Could you check a few things on this model? Use its own coordinates, in mm. Give positions to 0.01 mm unless a question says otherwise; leave off trailing zeros. Write each loop counter-clockwise with the first axis right and the second up, starting at its lowest first coordinate (ties: lowest second). Pieces come first, ordered by that corner, then holes. Notation, with made-up numbers: M -21,29 L -9,29 A27 ccw -9,61 Z; hole C -15.75,61 d1. An arc over 180 degrees is marked long. Use one line per item in the form item = value.
from build123d import *

# Parameters (mm, degrees)
LOFT_START          = -25
LOFT_1_OUTLINE_W    = 40
LOFT_1_OUTLINE_H    = 40
LOFT_1_DEPTH        = 10.8
SKETCH_1_R          = 1.5
CUT_EXTRUDE_1_DEPTH = 25


# Read off the part's stored shape, not the designer's step: По сечениям1
with BuildPart() as part:
    # По сечениям1 outline → По сечениям1 (new body)
    with BuildSketch(Plane.XY.offset(LOFT_START)):
        with Locations((-27.5, -27.5)):
            Rectangle(LOFT_1_OUTLINE_W, LOFT_1_OUTLINE_H)
    extrude(amount=LOFT_1_DEPTH)

    # Эскиз1 → Вырез-Вытянуть1 (cut)
    with BuildSketch(Plane.XY.offset(-14.2)):
        with Locations((-43.5, -11.5)):
            Circle(SKETCH_1_R)
        with Locations(Location((-43.5, -43.5, 0), (0, 0, 180))):
            Circle(SKETCH_1_R)
        with Locations(Location((-11.5, -11.5, 0), (0, 0, 180))):
            Circle(SKETCH_1_R)
        with Locations((-11.5, -43.5)):
            Circle(SKETCH_1_R)
    extrude(amount=-CUT_EXTRUDE_1_DEPTH, mode=Mode.SUBTRACT)


solid = part.part
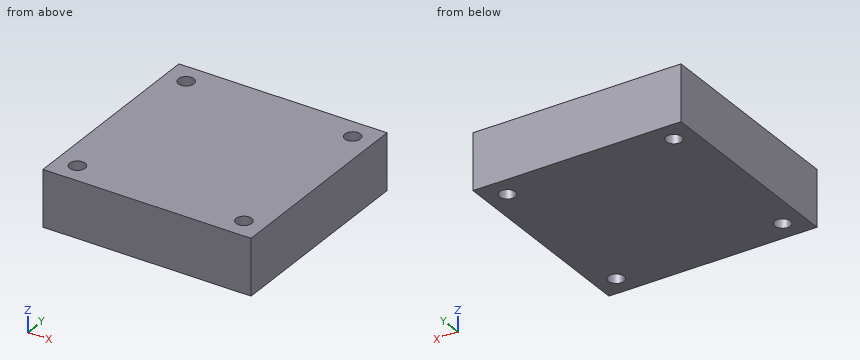
1) For pin 1 Ø5 at (x, y) = (-11.5, -11.5) entering from -Z; pin 2 Ø1.8 at (x, y) = (-43.5, -11.5) entering from +Z, each with a flat end and sliding along its axis, tell me the tip position at first contact or that it passes through.
Checked values:
pin_1 = -25
pin_2 = through
2) I want a section at A-A, the plane x = -43.5. Please give me the cut outline in (y, z).
Checked values:
outline = M -47.5,-25 L -45,-25 L -45,-14.2 L -47.5,-14.2 Z; M -42,-25 L -13,-25 L -13,-14.2 L -42,-14.2 Z; M -10,-25 L -7.5,-25 L -7.5,-14.2 L -10,-14.2 Z
3) I want a section at C-C, the plane z = -15.75. Please give me the cut outline in (x, y).
Checked values:
outline = M -47.5,-47.5 L -7.5,-47.5 L -7.5,-7.5 L -47.5,-7.5 Z; hole C -43.5,-43.5 d3; hole C -43.5,-11.5 d3; hole C -11.5,-43.5 d3; hole C -11.5,-11.5 d3
4) If I drill on L1, parallel to Y at x = -11.5, z = -20.75; L2, parallel to Y at x = -11, z = -24.25, over which ranges is the centre line in solid material (lowest first)?
Checked values:
L1 = -47.5 to -45, -42 to -13, -10 to -7.5
L2 = -47.5 to -44.91, -42.09 to -12.91, -10.09 to -7.5
